Geometry: see drawing. Coordinates: mm, zero at the bounding-box minimum. A direction names the side the tool comes from. Coordinates: 2 decimals unless noted, no trailing zeros. Write each loop counter-clockwise with the first axis right and the second up, starting at its lowest first coordinate (ties: lowest second). Pieces come first, ordered by that corner, then holes. Notation, with made-up numbers: (68.25, -11.75) - (87.25, -11.75) arc R19 ccw to (87.25, 23.25) - close; hole circle Ø6 at (-23, 22.5). An arc over 180 degrees is marked (long way). Use a Markdown table: item, result. Add a question column.
Q1. Pin query (flat end, axial travel): P1, Ø5, axis at x = 8, z = 49.5, coming from the -Y side; P2, Ø5, axis at x = 1, z = 63.5, coming from the -Y side; P3, Ø1, axis at x = 8, z = 19, coming from the +Y side (1 decimal). Return the tip coordinate at first contact, or that it passes through.
Q2. Section query C-C (y = 20). Return the cut outline in (x, z), then the cut area to 3 significant figures.
Q3. Section query B-B (z = 24). Return the cut outline in (x, y).
Q4. Section query A-A (x = 7.5). Give the number of separate pieces and of enclosed holes in the cut face.
Q5. Material intervals for probe 1 along Z at (x, y) = (3.25, 16.5) (1 decimal); probe 2 along Y at (x, z) = (1.25, 66) (1 decimal); probe 3 along Y at (x, z) = (4.25, 22.5) (1 decimal), sorted ascending. Write a range as from..to.
Q6. Set-up query: the marked faces 1 and 2. Return all of +Z, -Z, +X, -X, +Y, -Y with unobstructed straight access to the full face (end or side cutting, diameter ignored); none if empty.
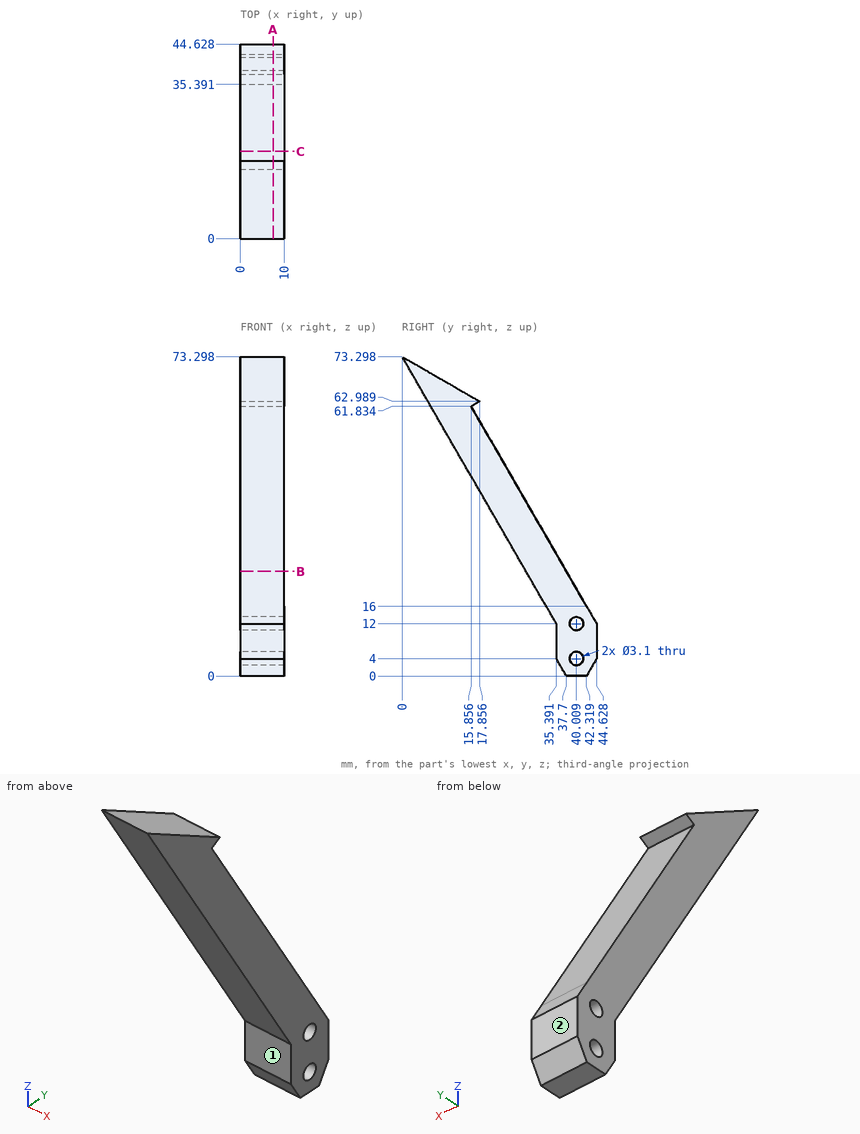
Values follow:
| question | item | result |
|---|---|---|
| 1 | P1 | y = 12.3 |
| 1 | P2 | y = 4.21 |
| 1 | P3 | y = 40.9 |
| 2 | outline | (0, 38.66) - (10, 38.66) - (10, 54.66) - (0, 54.66) - close |
| 2 | area | 160 mm2 |
| 3 | outline | (0, 28.46) - (10, 28.46) - (10, 37.7) - (0, 37.7) - close |
| 4 | separate pieces | 1 |
| 4 | enclosed holes | 2 |
| 5 | probe 1 | 44.7..60.7, 62.2..63.8 |
| 5 | probe 2 | 4.2..12.6 |
| 5 | probe 3 | 29.3..38.6 |
| 6 | face 1 | -Z, +X, -X, -Y |
| 6 | face 2 | +Z, -Z, +X, -X, +Y |
